Source: CAD feature listing. Evaluate the final solid. Frame: model axes, mm. Face numbers are marked on the shaded views. A direction names the side the tool comes from. Round coordinates to 2 decimals unless told otherwise and drop trailing zeros. Loops run counter-clockwise (first coordinate to the right, second up) from the corner with the lowest first, then second, coordinate; pieces in that order, holes last. Notation, with made-up numbers: M 12,64 L 23,64 A24 ccw 23,74 Z; hole C 9.5,25.5 d8. An arc over 180 degrees is marked long. Write each question's results on one line, items separated by ' | '. Start each with the question number.
1. Ray query, line 1 (Z direction, x = -5.75, y = 0) (3 decimals); line 2 (Z direction, x = -8, y = 0) (3 decimals); line 3 (Y direction, x = -7, z = 38). Return the intervals inside material, ascending.
2. Set-up query: the marked faces 1, 2, 3 and 4. Return all of +Z, -Z, +X, -X, +Y, -Y with unobstructed straight access to the full face (end or side cutting, diameter ignored); none if empty.
3. Section D-D on x = -118. Output: boundary loops of the cut face in (y, z) (3 decimals), and give its area (3 significant figures).
4. Section C-C on y = 0. Output: boundary loops of the cut face in (x, z) (3 decimals).
5. Draft query along X for the marked faces 5, 6, 7 and 8. Return one class per face: released by +X, released by -X, zero draft, split by the parting line, or undercut.
6. Contact query for flat-ended pins moving along their axis: pin 1 Ø14 at (x, y) = (-109, -2) entering from -Z; pin 2 Ø2 at (x, y) = (-142.5, 6.5) entering from +Z; pin 3 Ø15 at (x, z) = (-99.5, -4.5) entering from +Y; pin 4 Ø3 at (x, z) = (-29, 26) entering from +Y. Output: stop coordinate, or through.
7. Section B-B on y = -10.75. Output: boundary loops of the cut face in (x, z) (3 decimals).
8. Section A-A on z = 0. Output: boundary loops of the cut face in (x, y) (3 decimals).
from build123d import *

# Parameters (mm, degrees)
F1_DEPTH  = 6.35
F3_DEPTH  = 3.175
F5_DEPTH  = 3.175
F6_R      = 15.875
F7_DEPTH  = 12.7
F9_DEPTH  = 12.7
F11_DEPTH = 25.401
F12_R     = 12.7
F13_DEPTH = 25.401
F14_R     = 3.175
F15_DEPTH = 180.976


with BuildPart() as f1:
    # F0 (on Front) → F1 (new body, symmetric)
    with BuildSketch(Plane.XZ):
        with BuildLine():
            ThreePointArc((0, -25.4), (-25.4, 0), (0, 25.4))
            Line((0, 25.4), (0, 44.45))
            Line((0, 44.45), (-12.7, 44.45))
            Line((-12.7, 44.45), (-12.7, 31.75))
            Line((-12.7, 31.75), (-19.05, 31.75))
            ThreePointArc((-19.05, 31.75), (-36.7086920337, 17.7094988016), (-58.7057372898, 12.7))
            Line((-58.7057372898, 12.7), (-149.225, 12.7))
            ThreePointArc((-149.225, 12.7), (-154.2063498325, 13.1932508375), (-158.9942307692, 14.6538461538))
            ThreePointArc((-158.9942307692, 14.6538461538), (-180.975, 0), (-158.9942307692, -14.6538461538))
            ThreePointArc((-158.9942307692, -14.6538461538), (-154.2063498325, -13.1932508375), (-149.225, -12.7))
            Line((-149.225, -12.7), (-58.7057372898, -12.7))
            ThreePointArc((-58.7057372898, -12.7), (-36.7086920337, -17.7094988016), (-19.05, -31.75))
            Line((-19.05, -31.75), (-12.7, -31.75))
            Line((-12.7, -31.75), (-12.7, -44.45))
            Line((-12.7, -44.45), (0, -44.45))
            Line((0, -44.45), (0, -25.4))
        make_face()
    extrude(amount=F1_DEPTH, both=True)

    # F2 (on face) → F3 (cut)
    with BuildSketch(Plane.XZ.offset(6.35)):
        with BuildLine():
            ThreePointArc((-127, 9.525), (-136.525, 0), (-127, -9.525))
            Line((-127, -9.525), (-50.8, -9.525))
            ThreePointArc((-50.8, -9.525), (-41.275, 0), (-50.8, 9.525))
            Line((-50.8, 9.525), (-127, 9.525))
        make_face()
    extrude(amount=-F3_DEPTH, mode=Mode.SUBTRACT)

    # F4 (on face) → F5 (cut)
    with BuildSketch(Plane(origin=(0, 6.35, 0), x_dir=(-1, 0, 0), z_dir=(0, 1, 0))):
        with BuildLine():
            ThreePointArc((50.8, 9.525), (41.275, 0), (50.8, -9.525))
            Line((50.8, -9.525), (127, -9.525))
            ThreePointArc((127, -9.525), (136.525, 0), (127, 9.525))
            Line((127, 9.525), (50.8, 9.525))
        make_face()
    extrude(amount=-F5_DEPTH, mode=Mode.SUBTRACT)

    # F6 (on Front) → F7 (join, symmetric)
    with BuildSketch(Plane.XZ):
        with Locations((-165.1, 0)):
            Circle(F6_R)
    extrude(amount=F7_DEPTH, both=True)

    # F8 (on Front) → F9 (join, symmetric)
    with BuildSketch(Plane.XZ):
        with BuildLine():
            Line((0, -31.75), (0, 31.75))
            ThreePointArc((0, 31.75), (-31.75, 0), (0, -31.75))
        make_face()
    extrude(amount=F9_DEPTH, both=True)

    # F10 (on face) → F11 (cut, through all)
    with BuildSketch(Plane.XZ.offset(12.7)):
        with BuildLine():
            Line((0, -25.4), (0, 25.4))
            ThreePointArc((0, 25.4), (-25.4, 0), (0, -25.4))
        make_face()
    extrude(amount=-F11_DEPTH, mode=Mode.SUBTRACT)

    # F12 (on face) → F13 (cut, through all)
    with BuildSketch(Plane.XZ.offset(12.7)):
        with Locations((-165.1, 0)):
            Circle(F12_R)
    extrude(amount=-F13_DEPTH, mode=Mode.SUBTRACT)

    # F14 (on Right) → F15 (cut, through all)
    with BuildSketch(Plane.YZ):
        with Locations((0, 38.1)):
            Circle(F14_R)
        with Locations((0, -38.1)):
            Circle(F14_R)
    extrude(amount=-F15_DEPTH, mode=Mode.SUBTRACT)


solid = f1.part
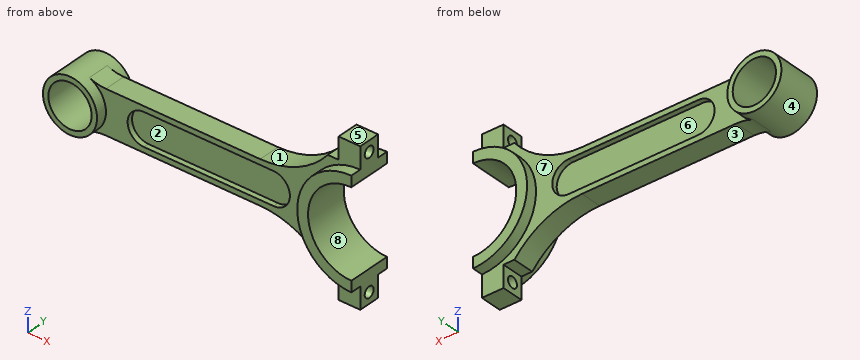
Taken from the geometry:
1) line 1: -44.45 to -41.275, -34.925 to -24.741, 24.741 to 34.925, 41.275 to 44.45 | line 2: -44.45 to -41.275, -34.925 to -24.107, 24.107 to 34.925, 41.275 to 44.45 | line 3: -6.35 to -3.17, 3.17 to 6.35
2) face 1: +Z, +Y, -Y | face 2: -Y | face 3: -Z, +Y, -Y | face 4: none
3) outline: M -6.35,-12.7 L 6.35,-12.7 L 6.35,-9.525 L 3.175,-9.525 L 3.175,9.525 L 6.35,9.525 L 6.35,12.7 L -6.35,12.7 L -6.35,9.525 L -3.175,9.525 L -3.175,-9.525 L -6.35,-9.525 Z | area: 202 mm^2
4) outline: M -158.994,-14.654 A25.4 cw -149.225,-12.7 L -58.706,-12.7 A50.8 cw -19.05,-31.75 L -12.7,-31.75 L -12.7,-34.925 L 0,-34.925 L 0,-25.4 A25.4 cw 0,25.4 L 0,34.925 L -12.7,34.925 L -12.7,31.75 L -19.05,31.75 A50.8 cw -58.706,12.7 L -149.225,12.7 A25.4 cw -158.994,14.654 A15.875 ccw long Z; M -12.7,-44.45 L 0,-44.45 L 0,-41.275 L -12.7,-41.275 Z; M -12.7,41.275 L 0,41.275 L 0,44.45 L -12.7,44.45 Z; hole C -165.1,0 d25.4
5) face 5: zero draft | face 6: undercut | face 7: undercut | face 8: released by +X
6) pin 1: z = -12.7 | pin 2: z = 12.7 | pin 3: y = 6.35 | pin 4: through
7) outline: C -165.1,0 d31.75; M 0,-31.75 L 0,-25.4 A25.4 cw 0,25.4 L 0,31.75 A31.75 ccw Z; hole C -165.1,0 d25.4
8) outline: M -180.975,-12.7 L -177.8,-12.7 L -177.8,12.7 L -180.975,12.7 Z; M -152.4,-12.7 L -149.225,-12.7 L -149.225,-6.35 L -136.525,-6.35 L -136.525,-3.175 L -41.275,-3.175 L -41.275,-6.35 L -31.75,-6.35 L -31.75,-12.7 L -25.4,-12.7 L -25.4,12.7 L -31.75,12.7 L -31.75,6.35 L -41.275,6.35 L -41.275,3.175 L -136.525,3.175 L -136.525,6.35 L -149.225,6.35 L -149.225,12.7 L -152.4,12.7 Z
